```python
from build123d import *

# Parameters (mm, degrees)
SZKIC1_R                    = 75
DODANIE_WYCI_GNI_CIE1_DEPTH = 40
SZKIC2_R                    = 6
WYTNIJ_WYCI_GNI_CIE1_DEPTH  = 40
SZKIC3_R                    = 47.5
WYTNIJ_WYCI_GNI_CIE2_DEPTH  = 40
SZKIC4_W                    = 50
SZKIC4_H                    = 20
DODANIE_WYCI_GNI_CIE2_DEPTH = 100
SZKIC6_W                    = 50
SZKIC6_H                    = 49.999779654
DODANIE_WYCI_GNI_CIE3_DEPTH = 20
SZKIC7_R                    = 7
WYTNIJ_WYCI_GNI_CIE3_DEPTH  = 226
ZAOKR_GLENIE1_R             = 10
ZAOKR_GLENIE2_R             = 10
DODANIE_WYCI_GNI_CIE4_DEPTH = 100
SZKIC10_W                   = 50
SZKIC10_H                   = 50
DODANIE_WYCI_GNI_CIE5_DEPTH = 100
SZKIC12_R                   = 7
WYTNIJ_WYCI_GNI_CIE5_DEPTH  = 163.5
WYTNIJ_WYCI_GNI_CIE6_DEPTH  = 161


with BuildPart() as part:
    # Szkic1 → Dodanie-wyciągnięcie1 (new body)
    with BuildSketch(Plane.XY):
        Circle(SZKIC1_R)
    extrude(amount=DODANIE_WYCI_GNI_CIE1_DEPTH)

    # Szkic2 → Wytnij-wyciągnięcie1 (cut)
    with BuildSketch(Plane.XY.offset(40)):
        with Locations((-55, 0)):
            Circle(SZKIC2_R)
        with Locations((0, 55)):
            Circle(SZKIC2_R)
        with Locations((55, 0)):
            Circle(SZKIC2_R)
        with Locations((0, -55)):
            Circle(SZKIC2_R)
    extrude(amount=-WYTNIJ_WYCI_GNI_CIE1_DEPTH, mode=Mode.SUBTRACT)

    # Szkic3 → Wytnij-wyciągnięcie2 (cut)
    with BuildSketch(Plane.XY.offset(40)):
        Circle(SZKIC3_R)
    extrude(amount=-WYTNIJ_WYCI_GNI_CIE2_DEPTH, mode=Mode.SUBTRACT)

    # Szkic4 → Dodanie-wyciągnięcie2 (add, symmetric)
    with BuildSketch(Plane(origin=(0, 0, 0), x_dir=(-0.707106781, -0.707106781, 0), z_dir=(0.707106781, -0.707106781, 0))):
        with Locations((0, 10)):
            Rectangle(SZKIC4_W, SZKIC4_H)
    extrude(amount=DODANIE_WYCI_GNI_CIE2_DEPTH, both=True)

    # Szkic6 → Dodanie-wyciągnięcie3 (add)
    with BuildSketch(Plane(origin=(70.710678119, -70.710678119, 0), x_dir=(0, 0, -1), z_dir=(0.707106781, -0.707106781, 0))):
        with Locations((45, 0.000110173)):
            Rectangle(SZKIC6_W, SZKIC6_H)
    dodanie_wyci_gni_cie3 = extrude(amount=-DODANIE_WYCI_GNI_CIE3_DEPTH)

    # Lustro1: Dodanie-wyciągnięcie3 across plane
    add(dodanie_wyci_gni_cie3.mirror(Plane(origin=(0, 0, 0), x_dir=(0, 0, 1), z_dir=(0.707106781, -0.707106781, 0))))

    # Szkic7 → Wytnij-wyciągnięcie3 (cut, through all)
    with BuildSketch(Plane(origin=(-70.710678119, 70.710678119, 0), x_dir=(0, 0, 1), z_dir=(-0.707106781, 0.707106781, 0))):
        with Locations((-45, 0)):
            Circle(SZKIC7_R)
    extrude(amount=-WYTNIJ_WYCI_GNI_CIE3_DEPTH, mode=Mode.SUBTRACT)

    # Zaokrąglenie1
    zaokr_glenie1_edges = [part.edges().sort_by_distance(p)[0] for p in [
        (81.317279836, -45.961940777, -70),
        (45.962096585, -81.317124028, -70),
        (-81.317124028, 45.962096585, -70),
        (-45.961940777, 81.317279836, -70),
    ]]
    fillet(zaokr_glenie1_edges, radius=ZAOKR_GLENIE1_R)

    # Zaokrąglenie2
    zaokr_glenie2_edges = [part.edges().sort_by_distance(p)[0] for p in [
        (-70.710678119, 70.710678119, 0),
        (70.710678119, -70.710678119, 0),
    ]]
    fillet(zaokr_glenie2_edges, radius=ZAOKR_GLENIE2_R)

    # Szkic8 → Dodanie-wyciągnięcie4 (add)
    with BuildSketch(Plane(origin=(0, 0, -20), x_dir=(-1, 0, 0), z_dir=(0, 0, -1))):
        Polygon((0, 35.355339059), (35.355339059, 0), (0, -35.355339059), (-35.355339059, 0), align=None)
    extrude(amount=DODANIE_WYCI_GNI_CIE4_DEPTH)

    # Szkic10 → Dodanie-wyciągnięcie5 (add)
    with BuildSketch(Plane(origin=(17.67766953, 17.67766953, 0), x_dir=(0, 0, -1), z_dir=(0.707106781, 0.707106781, 0))):
        with Locations((95, 0)):
            Rectangle(SZKIC10_W, SZKIC10_H)
    extrude(amount=DODANIE_WYCI_GNI_CIE5_DEPTH)

    # Szkic12 → Wytnij-wyciągnięcie5 (cut, through all)
    with BuildSketch(Plane(origin=(17.67766953, -17.67766953, 0), x_dir=(0, 0, -1), z_dir=(0.707106781, -0.707106781, 0))):
        with Locations((95, 105)):
            Circle(SZKIC12_R)
    extrude(amount=-WYTNIJ_WYCI_GNI_CIE5_DEPTH, mode=Mode.SUBTRACT)

    # Szkic14 → Wytnij-wyciągnięcie6 (cut, through all)
    with BuildSketch(Plane(origin=(0, 0, -120), x_dir=(-1, 0, 0), z_dir=(0, 0, -1))):
        with BuildLine():
            Line((-80.610173055, 60.811183182), (-98.287842585, 78.488852712))
            Line((-98.287842585, 78.488852712), (-78.488852712, 98.287842585))
            Line((-78.488852712, 98.287842585), (-60.811183182, 80.610173055))
            ThreePointArc((-60.811183182, 80.610173055), (-60.811183182, 60.811183182), (-80.610173055, 60.811183182))
        make_face()
    extrude(amount=-WYTNIJ_WYCI_GNI_CIE6_DEPTH, mode=Mode.SUBTRACT)


solid = part.part
```
Source: CAD feature listing. Evaluate the final solid. Frame: model axes, mm. A direction names the side the tool comes from. Give positions to 0.01 mm unless a question says otherwise; leave off trailing zeros. Loops run counter-clockwise (first coordinate to the right, second up) from the corner with the lowest first, then second, coordinate; pieces in that order, holes last. Notation, with made-up numbers: (12.5, 73.5) - (64.5, 73.5) arc R32 cw to (64.5, 107.5) - close; hole circle Ø10 at (72, 35). An arc over 180 degrees is marked (long way). Use CSV: the item, a comma, the result in double quotes.
1) Cut plane A-A (z = -57). Output: boundary loops of the cut face in (x, y), and give its area (3 significant figures).
Worked out:
outline,"(-88.39, 53.03) - (-74.25, 38.89) - (-38.89, 74.25) - (-53.03, 88.39) - close; (-35.36, 0) - (0, -35.36) - (35.36, 0) - (0, 35.36) - close; (38.89, -74.25) - (53.03, -88.39) - (88.39, -53.03) - (74.25, -38.89) - close"
area,"4,500 mm^2"
2) Pin query (flat end, axial travel): P1, Ø3, axis at y = 10, z = -63, coming from the +X side; P2, Ø10.5, axis at x = -69, y = 63, coming from the -Z side; P3, Ø12, axis at x = 52, z = -74.5, coming from the +Y side; P4, Ø12, axis at x = -15, y = -38.5, coming from the +Z side. Return the tip coordinate at first contact, or that it passes through.
Worked out:
P1,"stops at x = 26.86"
P2,"stops at z = -70"
P3,"stops at y = 93.36"
P4,"passes through"
3) Cut plane B-B (y = -21). Output: boundary loops of the cut face in (x, z), and give its area (3 significant figures).
Worked out:
outline,"(-72, 0) - (-42.61, 0) - (-42.61, 40) - (-72, 40) - close; (-14.36, -120) - (14.36, -120) - (14.36, -20) - (56.36, -20) - (56.36, 0) - (72, 0) - (72, 40) - (42.61, 40) - (42.61, 0) - (-14.36, 0) - close"
area,"6,640 mm^2"
4) Mould query, pull axis X, two halves, no side actions, for faces 5 (the flat face through (89.3, 69.5, -95.4)), 6 (the cylindrical face through (68.45, -68.94, -3.01)), 7 (the flat face through (5.15, 40.505, -80.411)). Classes: +X half, -X half, draft (parallel to the pull), parting line (faces both ways), or undercut.
Worked out:
face 5,"undercut"
face 6,"+X half"
face 7,"-X half"
5) Cut plane C-C (x = -16.5). Output: boundary loops of the cut face in (y, z).
Worked out:
outline,"(-73.16, 0) - (-44.54, 0) - (-44.54, 40) - (-73.16, 40) - close; (-18.86, -120) - (18.86, -120) - (18.86, -20) - (51.86, -20) - (51.86, 0) - (73.16, 0) - (73.16, 40) - (44.54, 40) - (44.54, 0) - (-18.86, 0) - close"
6) Line query: line 1 (Y direction, x = 0, z = 13.5); line 2 (Z direction, x = 25.5, y = 7); line 3 (Z direction, x = 39.5, y = -33.5). Output: solid intervals per line, ascending.
Worked out:
line 1,"y = -75 to -61, -49 to -47.5, 47.5 to 49, 61 to 75"
line 2,"z = -120 to 0"
line 3,"z = -20 to 40"
7) Set-up query: faces 1 (the flat face through (52.888, -60.249, -39.094)), 2 (the cylindrical face through (-10.3, -46.37, 20.28)), 3 (the flat face through (-64, 64, -70)), 4 (the flat face through (-58, 58, 0)). Return all of +Z, -Z, +X, -X, +Y, -Y with unobstructed straight access to the full face (end or side cutting, diameter ignored); none if empty.
Worked out:
face 1,"-Z, -X, +Y"
face 2,"+Z"
face 3,"-Z, -X, +Y, -Y"
face 4,"+Z, -X, +Y"
